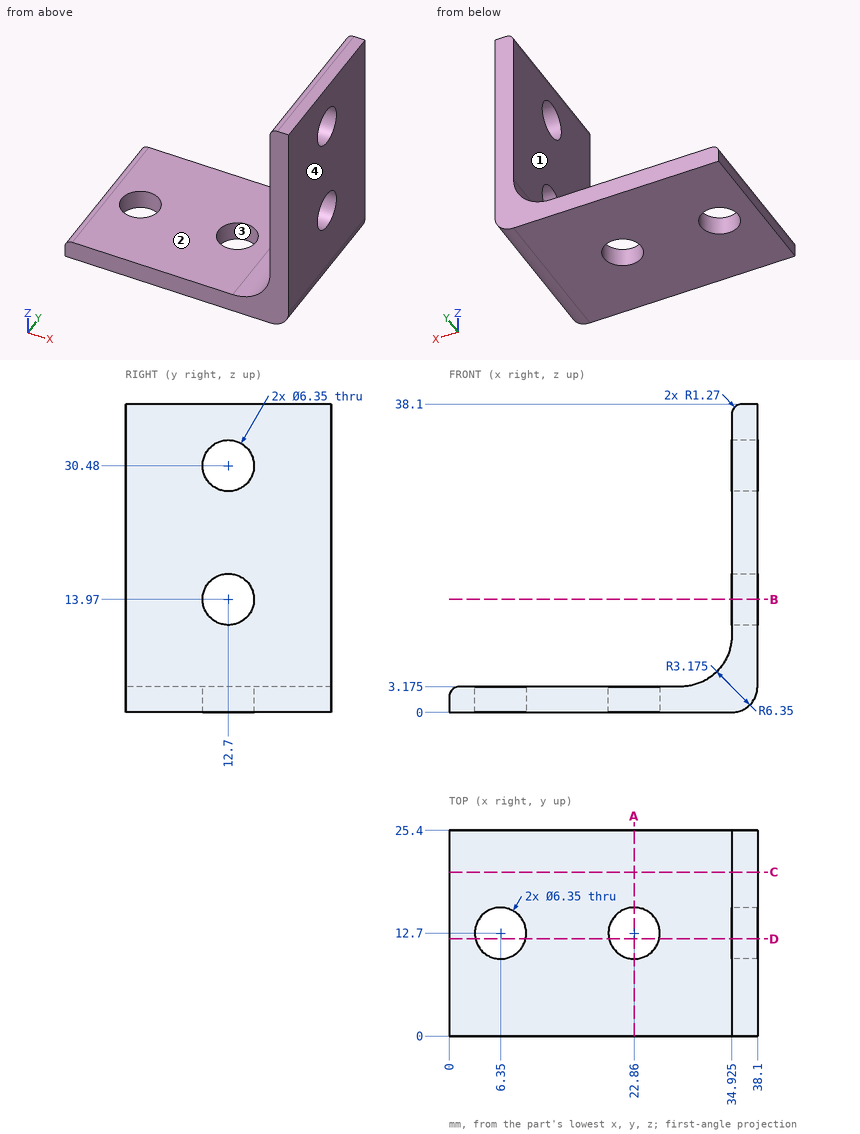
Here's the drawing with two shaded views (mm, measured from the low corner). I have some questions. Give positions to 0.01 mm unless a question says otherwise; leave off trailing zeros. Order: outer loops, then holes, each group sorted by start corner. A loop starts at its lowest first (then second) coordinate and runs counter-clockwise, first axis right, second up. Notation, with made-up numbers: M 63.5,-14.75 L 108.5,-14.75 A11 ccw 108.5,0.25 Z; hole C 37,16.25 d7. An arc over 180 degrees is marked long. One line per question, with ' | ' between items.
Item 1: Suppose I cut it at A-A, the plane x = 22.86. Write out the boundary of the cut face in (y, z) (3 decimals), then the cut area to 3 significant figures.
Answer block:
outline: M 0,0 L 9.525,0 L 9.525,3.175 L 0,3.175 Z; M 15.875,0 L 25.4,0 L 25.4,3.175 L 15.875,3.175 Z | area: 60.5 mm2
Item 2: We'd pull the mould along X, two halves only. Please class the marked faces 1, 2, 3 and 4: released by +X, released by -X, zero draft, split by the parting line, or undercut.
Answer block:
face 1: released by -X | face 2: zero draft | face 3: undercut | face 4: released by +X
Item 3: Suppose I cut it at D-D, the plane y = 12. Write out the boundary of the cut face in (x, z) (3 decimals), then the cut area to 3 significant figures.
Answer block:
outline: M 0,0 L 3.253,0 L 3.253,3.175 L 1.27,3.175 A1.27 ccw 0,1.905 Z; M 9.447,0 L 19.763,0 L 19.763,3.175 L 9.447,3.175 Z; M 25.957,0 L 34.925,0 A3.175 ccw 38.1,3.175 L 38.1,10.873 L 34.925,10.873 L 34.925,9.525 A6.35 cw 28.575,3.175 L 25.957,3.175 Z; M 34.925,17.067 L 38.1,17.067 L 38.1,27.383 L 34.925,27.383 Z; M 34.925,33.577 L 38.1,33.577 L 38.1,38.1 L 36.195,38.1 A1.27 ccw 34.925,36.83 Z | area: 159 mm2
Item 4: I'm going to push flat-ended pins straight in: pin 1 Ø7.5 at (y, z) = (12.7, 30.48) entering from -X (3 decimals); pin 2 Ø10 at (x, y) = (22.86, 12.7) entering from +Z (3 decimals); pin 3 Ø4 at (x, y) = (31, 10) entering from +Z. Where does each tip first touch, or does it pass through?
Answer block:
pin 1: stops at x = 34.925 | pin 2: stops at z = 3.175 | pin 3: stops at z = 4.97
Item 5: Please list where these lines run through material, in increasing order: L1, parallel to Y at x = 6.35, z = 0.95 (3 decimals); L2, parallel to X at y = 1.25, z = 35 (3 decimals); L3, parallel to Z at x = 27, y = 5.5 (3 decimals).
Answer block:
L1: y = 0 to 9.525, 15.875 to 25.4 | L2: x = 34.925 to 38.1 | L3: z = 0 to 3.175
Item 6: Suppose I cut it at B-B, the plane z = 13.97. Write out the boundary of the cut face in (x, y) (3 decimals).
Answer block:
outline: M 34.925,0 L 38.1,0 L 38.1,9.525 L 34.925,9.525 Z; M 34.925,15.875 L 38.1,15.875 L 38.1,25.4 L 34.925,25.4 Z
Item 7: Suppose I cut it at C-C, the plane y = 20.25. Write out the boundary of the cut face in (x, z) (3 decimals), then the cut area to 3 significant figures.
Answer block:
outline: M 0,0 L 34.925,0 A3.175 ccw 38.1,3.175 L 38.1,38.1 L 36.195,38.1 A1.27 ccw 34.925,36.83 L 34.925,9.525 A6.35 cw 28.575,3.175 L 1.27,3.175 A1.27 ccw 0,1.905 Z | area: 238 mm2
